The listing builds one solid part. Answer for the finished solid, in the listing's coordinates (mm). A direction names the side the tool comes from. Coordinates: 2 decimals unless noted, no trailing zeros. Write each loop counter-clockwise with the first axis right and the second up, starting at its lowest first coordinate (ties: lowest second). Pieces come first, ordered by that corner, then holes.
from build123d import *

# Parameters (mm, degrees)
SKETCH1_W           = 45
SKETCH1_H           = 7.5
SKETCH1_H_2         = 12.5
BOSS_EXTRUDE1_DEPTH = 2
BOSS_EXTRUDE2_DEPTH = 8.25
SKETCH3_W           = 10
SKETCH3_H           = 5
BOSS_EXTRUDE3_DEPTH = 3
SKETCH4_W           = 40
SKETCH4_H           = 1
CUT_EXTRUDE1_DEPTH  = 2
LOFT2_START         = -7.5
LOFT2_DEPTH         = 15


# Read off the part's stored shape, not the designer's step: Loft2
with BuildPart() as part:
    # Sketch1 → Boss-Extrude1 (new body)
    with BuildSketch(Plane.XY):
        with Locations((0, 6.25)):
            Rectangle(SKETCH1_W, SKETCH1_H)
        with Locations((0, -3.75)):
            Rectangle(SKETCH1_W, SKETCH1_H_2)
    extrude(amount=BOSS_EXTRUDE1_DEPTH)

    # Sketch1<3> → Boss-Extrude2 (add)
    with BuildSketch(Plane.XY):
        Polygon((-22.5, 2.5), (-24.5, 2.5), (-24.5, -12), (24.5, -12), (24.5, 2.5), (22.5, 2.5), (22.5, -10), (-22.5, -10), align=None)
    extrude(amount=BOSS_EXTRUDE2_DEPTH)

    # Sketch3 → Boss-Extrude3 (add)
    with BuildSketch(Plane.XY.offset(8.25)):
        with Locations((-19.5, 0)):
            Rectangle(SKETCH3_W, SKETCH3_H)
        with Locations((19.5, 0)):
            Rectangle(SKETCH3_W, SKETCH3_H)
    extrude(amount=BOSS_EXTRUDE3_DEPTH)

    # Sketch4 → Cut-Extrude1 (cut)
    with BuildSketch(Plane(origin=(0, 10, 0), x_dir=(1, 0, 0), z_dir=(0, 1, 0))):
        with Locations((0, -1)):
            Rectangle(SKETCH4_W, SKETCH4_H)
    extrude(amount=-CUT_EXTRUDE1_DEPTH, mode=Mode.SUBTRACT)

    # Loft2 outline → Loft2 (add)
    with BuildSketch(Plane.YZ.offset(LOFT2_START)):
        with BuildLine():
            add(Edge.make_bspline(
                [(1.5, 0), (1.5, -1.699673171), (2, -3.349836586), (2.5, -5)],
                knots=[0, 0, 0, 0, 1, 1, 1, 1], degree=3))
            Line((1.5, 0), (-1.5, 0))
            add(Edge.make_bspline(
                [(-1.5, 0), (-1.5, -1.699673171), (-2, -3.349836586), (-2.5, -5)],
                knots=[0, 0, 0, 0, 1, 1, 1, 1], degree=3))
            Line((-2.5, -5), (2.5, -5))
        make_face()
    extrude(amount=LOFT2_DEPTH)


solid = part.part
Q1. The part is cut by section C-C, the plane y = -3. Write down the section's boundary in (x, z).
Answers below:
outline: (-24.5, 0) - (24.5, 0) - (24.5, 8.25) - (22.5, 8.25) - (22.5, 2) - (-22.5, 2) - (-22.5, 8.25) - (-24.5, 8.25) - close
Q2. Find the intervals of material crossed by probe 1 along X at (y, z) = (-4.5, 5); probe 2 along Z at (x, y) = (14, 5); probe 3 along X at (y, z) = (7.5, 1.5), in increasing order.
Answers below:
probe 1: x = -24.5 to -22.5, 22.5 to 24.5
probe 2: z = 0 to 2
probe 3: x = -22.5 to 22.5
Q3. The part is cut by section B-B, the plane x = 17.5. Write down the section's boundary in (y, z), then the cut area to 3 significant figures.
Answers below:
outline: (-12, 0) - (10, 0) - (10, 0.5) - (8, 0.5) - (8, 1.5) - (10, 1.5) - (10, 2) - (-10, 2) - (-10, 8.25) - (-12, 8.25) - close; (-2.5, 8.25) - (2.5, 8.25) - (2.5, 11.25) - (-2.5, 11.25) - close
area: 69.5 mm2
Q4. Given pin 1 (6.5 mm diameter, centred on x = 11.5, y = -0.5, fed in from -Z); pin 2 (6 mm diameter, centred on x = 2, y = -2.5, fed in from +Z); pin 3 (0.9 mm diameter, centred on x = -18.5, z = 10, fed in from -Y), each flat-ended and moving along its own axis, determine where each tip first touches the part or whether it passes through.
Answers below:
pin 1: stops at z = 0
pin 2: stops at z = 2
pin 3: stops at y = -2.5
Q5. The part is cut by section A-A, the plane z = 9.5. Write down the section's boundary in (x, y), then the cut area to 3 significant figures.
Answers below:
outline: (-24.5, -2.5) - (-14.5, -2.5) - (-14.5, 2.5) - (-24.5, 2.5) - close; (14.5, -2.5) - (24.5, -2.5) - (24.5, 2.5) - (14.5, 2.5) - close
area: 100 mm2
Q6. Determine the mould class of faces 1 (the face through (22.5, 6, 1)), 2 (the face through (19, 0, 11.25)), 3 (the face through (20, 9, 1)) for opening direction X: released by +X, released by -X, zero draft, split by the parting line, or undercut.
Answers below:
face 1: released by +X
face 2: zero draft
face 3: undercut
Q7. Which of the six approach directions +Z, -Z, +X, -X, +Y, -Y give full straight-line access (tool end or side, diameter ignored) to faces 4 (the face through (0, 9, 1.5)), 5 (the face through (14.5, 0, 10)), 6 (the face through (-23, 2.5, 8)), 7 (the face through (7.5, 0, -3))?
Answers below:
face 4: +Y
face 5: +Z, +Y, -Y
face 6: +Z, -X, +Y
face 7: -Z, +X, +Y, -Y
Q8. The part is cut by section D-D, the plane x = -21. Write down the section's boundary in (y, z).
Answers below:
outline: (-12, 0) - (10, 0) - (10, 2) - (-10, 2) - (-10, 8.25) - (-12, 8.25) - close; (-2.5, 8.25) - (2.5, 8.25) - (2.5, 11.25) - (-2.5, 11.25) - close
